Geometry check sheet. Reference: drawing and pictorial views, mm from the part's lowest x, y, z. A direction names the side the tool comes from. Coordinates: 2 decimals unless noted, no trailing zeros. Write each loop counter-clockwise with the first axis right and the second up, starting at its lowest first coordinate (ties: lowest second). Pieces come first, ordered by that corner, then holes. Notation, with made-up numbers: (10.25, 45.5) - (20.25, 45.5) arc R34 cw to (20.25, 78.5) - close; hole circle Ø8 at (85, 46). An arc over 180 degrees is marked (long way). Use one line per item in the form item = value. Start each with the question number.
(1) Material ranges on line 1 (Z direction, x = 20, y = 10.5); line 2 (X direction, y = 3.75, z = 9.75) (3 decimals); line 3 (Y direction, x = 18.75, z = 17), recorded low to high. Write a range as [from, to].
(2) Sectioned sample at D-D (y = 2). Record the cut outline in (x, z), and give its area (3 significant figures).
(3) Gauge pin test, flat ends, axial feed: pin 1 Ø1.5 at (x, y) = (12.5, 6) entering from -Z; pin 2 Ø4 at (x, z) = (7.7, 9.75) entering from +Y. Record the tip position at first contact, or that the pin passes through.
(4) Mould release check, pull along Z, two halves, no side actions. Record for the marked faces 3, 4, 5 and 6: released by +Z, released by -Z, zero draft, split by the parting line, or undercut.
(5) Sectioned sample at C-C (z = 9.75). Record the cut outline in (x, y), and give its area (3 significant figures).
(6) Tool access check on the marked faces 1 and 2. Record the directions out of +Z, -Z, +X, -X, +Y, -Y that give a thin tool (end or side, any length) a straight path to the whole face; none if there is none.
(7) Sectioned sample at A-A (x = 16.7). Record the cut outline in (y, z), and give its area (3 significant figures).
(8) Sectioned sample at B-B (y = 9). Record the cut outline in (x, z).
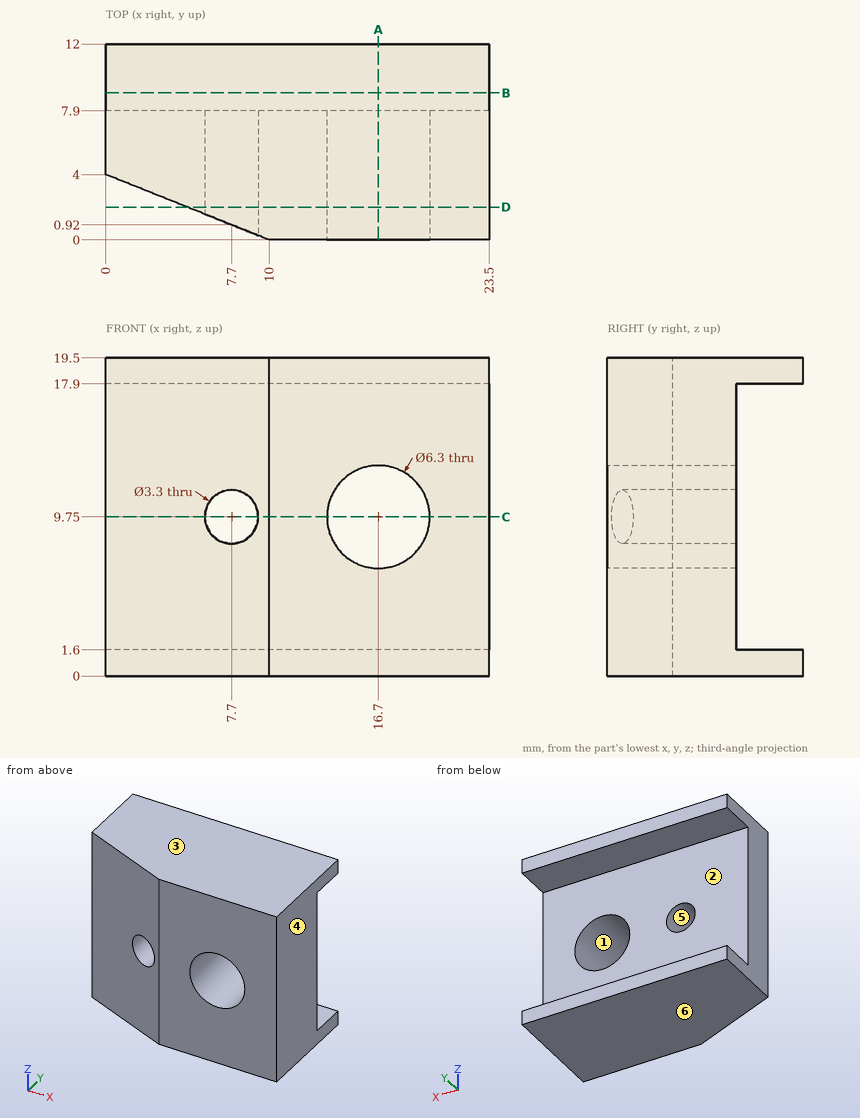
Answers below:
q1.line_1 = [0, 1.6], [17.9, 19.5]
q1.line_2 = [0.625, 6.05], [9.35, 13.55], [19.85, 23.5]
q1.line_3 = [0, 7.9]
q2.outline = (5, 0) - (23.5, 0) - (23.5, 19.5) - (5, 19.5) - close; hole circle Ø3.3 at (7.7, 9.75); hole circle Ø6.3 at (16.7, 9.75)
q2.area = 321 mm2
q3.pin_1 = 0
q3.pin_2 = 7.9
q4.face_3 = released by +Z
q4.face_4 = zero draft
q4.face_5 = undercut
q4.face_6 = released by -Z
q5.outline = (0, 4) - (6.05, 1.58) - (6.05, 7.9) - (0, 7.9) - close; (9.35, 0.26) - (10, 0) - (13.55, 0) - (13.55, 7.9) - (9.35, 7.9) - close; (19.85, 0) - (23.5, 0) - (23.5, 7.9) - (19.85, 7.9) - close
q5.area = 92.8 mm2
q6.face_1 = +Y, -Y
q6.face_2 = +X, -X, +Y
q7.outline = (0, 0) - (12, 0) - (12, 1.6) - (7.9, 1.6) - (7.9, 6.6) - (0, 6.6) - close; (0, 12.9) - (7.9, 12.9) - (7.9, 17.9) - (12, 17.9) - (12, 19.5) - (0, 19.5) - close
q7.area = 117 mm2
q8.outline = (0, 0) - (23.5, 0) - (23.5, 1.6) - (0, 1.6) - close; (0, 17.9) - (23.5, 17.9) - (23.5, 19.5) - (0, 19.5) - close
